Here's how the part is built. I have some questions about the finished solid (model axes, mm). A direction names the side the tool comes from. Round coordinates to 2 decimals unless told otherwise and drop trailing zeros. Order: outer loops, then holes, each group sorted by start corner. A loop starts at its lowest first (then second) coordinate and runs counter-clockwise, first axis right, second up. Notation, with made-up numbers: (-31, 22) -> (7, 22) arc R22 cw to (7, 42) -> close; hole circle Ø6 at (-31.5, 86.5). An arc over 180 degrees is marked (long way). One line per item, written item: value.
```python
from build123d import *

# Parameters (mm, degrees)
EXTRUDE1_DEPTH       = 39.5
SKETCH2_W            = 19.5
SKETCH2_H            = 8.1
EXTRUDE2_DEPTH       = 40.5
HOLEWZD1_D           = 8
HOLEWZD1_DEPTH       = 80.000025
HOLEWZD2_D           = 6.5
HOLEWZD2_CBORE_D     = 11
HOLEWZD2_CBORE_DEPTH = 4.4
FILLET1_R            = 1
FILLET2_R            = 3


with BuildPart() as part:
    # Sketch1 → Extrude1 (new body)
    with BuildSketch(Plane.XZ.offset(40)):
        with BuildLine():
            Line((-2, -8.1), (-2, -7.228416147))
            ThreePointArc((-2, -7.228416147), (5.968668193, 4.541475531), (-7.5, 0))
            Line((-7.5, 0), (-27.5, 0))
            Line((-27.5, 0), (-27.5, -8.1))
            Line((-27.5, -8.1), (-2, -8.1))
        make_face()
    extrude(amount=-EXTRUDE1_DEPTH)

    # Sketch2 → Extrude2 (add)
    with BuildSketch(Plane(origin=(0, -0.5, 0), x_dir=(-1, 0, 0), z_dir=(0, 1, 0))):
        with Locations((17.75, -4.05)):
            Rectangle(SKETCH2_W, SKETCH2_H)
    extrude(amount=EXTRUDE2_DEPTH)

    # HoleWzd1
    with Locations(Plane(origin=(0, -40, 0), x_dir=(-1, 0, 0), z_dir=(0, -1, 0))):
        with Locations((0, 0)):
            Hole(HOLEWZD1_D / 2, depth=HOLEWZD1_DEPTH)

    # HoleWzd2 (through all)
    with Locations(Plane.XY):
        with Locations((-15.5, -21.5), (-15.5, 21.5)):
            CounterBoreHole(HOLEWZD2_D / 2, HOLEWZD2_CBORE_D / 2, HOLEWZD2_CBORE_DEPTH)

    # Fillet1
    fillet1_edges = [part.edges().sort_by_distance(p)[0] for p in [
        (-27.5, 0, 0),
    ]]
    fillet(fillet1_edges, radius=FILLET1_R)

    # Fillet2
    # the kernel refuses this fillet: 3 mm, written as the material it takes off along each edge
    with BuildSketch(Plane(origin=(-27.5, -40, 6.5), x_dir=(1, 0, 0), z_dir=(0, 0, -1)), Plane(origin=(-27.5, 40, 6.5), x_dir=(0, -1, 0), z_dir=(0, 0, -1))) as fillet2_piece_1:
        with BuildLine():
            CenterArc((FILLET2_R, -FILLET2_R), FILLET2_R, 90, 90)
            Line((0, -FILLET2_R), (0, 0))
            Line((0, 0), (FILLET2_R, 0))
        make_face()
    extrude(amount=22.1, mode=Mode.SUBTRACT)


solid = part.part
```
Q1. Which directions (+Z, -Z, +X, -X, +Y, -Y) give clear straight access to the entire face, cutting with the end or side of a thin tool? Please do faces 1 (the face through (-12.543, 26.138, -2.169)), 2 (the face through (-8, 19, -4)), 3 (the face through (-17, -1, 0)), 4 (the face through (-16, 40, -4)).
Answers:
face 1: +Z
face 2: +Z, -Z, +X, +Y
face 3: +Z, -X, +Y, -Y
face 4: +Z, -Z, +X, -X, +Y
Q2. For P1, Ø1.5, axis at x = -20.5, y = 5.5, coming from the +Z side; P2, Ø3, axis at y = -15.5, z = 3.5, coming from the -X side; P3, Ø6, axis at x = -15.5, y = -21.5, coming from the +Z side; P4, Ø5.5, axis at x = -14.5, y = -24, coming from the +Z side, each with a flat end and sliding along its axis, tell me the tip position at first contact or that it passes through.
Answers:
P1: z = 0
P2: x = -7.23
P3: through
P4: z = -4.4
Q3. I need wall thicknesses on line 1 along Y through (x, z) = (-15.5, -2.95); line 2 along Z through (x, y) = (-11.5, -34.5); line 3 along Y through (x, z) = (-17.5, -6.25). Which ranges of each line are inside material? Lowest first, please.
Answers:
line 1: -40 to -27, -16 to 16, 27 to 40
line 2: -8.1 to 0
line 3: -40 to -24.06, -18.94 to 18.94, 24.06 to 40
Q4. I want a section at D-D on y = 21.5. Write out the boundary of the cut face in (x, z).
Answers:
outline: (-27.5, -8.1) -> (-18.75, -8.1) -> (-18.75, -4.4) -> (-21, -4.4) -> (-21, 0) -> (-26.5, 0) arc R1 ccw to (-27.5, -1) -> close; (-12.25, -8.1) -> (-8, -8.1) -> (-8, 0) -> (-10, 0) -> (-10, -4.4) -> (-12.25, -4.4) -> close
Q5. I want a section at C-C on z = -2.25. Write out the boundary of the cut face in (x, y).
Answers:
outline: (-27.5, -37) arc R3 ccw to (-24.5, -40) -> (-3.31, -40) -> (-3.31, -0.5) -> (-8, -0.5) -> (-8, 40) -> (-24.5, 40) arc R3 ccw to (-27.5, 37) -> close; (3.31, -40) -> (7.15, -40) -> (7.15, -0.5) -> (3.31, -0.5) -> close; hole circle Ø11 at (-15.5, -21.5); hole circle Ø11 at (-15.5, 21.5)
Q6. I want a section at A-A on y = -21.5. Write out the boundary of the cut face in (x, z), then the cut area to 3 significant figures.
Answers:
outline: (-27.5, -8.1) -> (-18.75, -8.1) -> (-18.75, -4.4) -> (-21, -4.4) -> (-21, 0) -> (-26.5, 0) arc R1 ccw to (-27.5, -1) -> close; (-12.25, -8.1) -> (-2, -8.1) -> (-2, -7.23) arc R7.5 ccw (long way) to (-7.5, 0) -> (-10, 0) -> (-10, -4.4) -> (-12.25, -4.4) -> close; hole circle Ø8 at (0, 0)
area: 231 mm2
Q7. I want a section at B-B on x = -15.5. Write out the boundary of the cut face in (y, z).
Answers:
outline: (-40, -8.1) -> (-24.75, -8.1) -> (-24.75, -4.4) -> (-27, -4.4) -> (-27, 0) -> (-40, 0) -> close; (-18.25, -8.1) -> (18.25, -8.1) -> (18.25, -4.4) -> (16, -4.4) -> (16, 0) -> (-16, 0) -> (-16, -4.4) -> (-18.25, -4.4) -> close; (24.75, -8.1) -> (40, -8.1) -> (40, 0) -> (27, 0) -> (27, -4.4) -> (24.75, -4.4) -> close
Q8. If we mould it in two halves opening along Y, with no side actions, what happens to faces 5 (the face through (-9, -40, -2)), 6 (the face through (-12.253, -21.357, -6.276)), 7 (the face through (-15, -1, -8.1))? For each: pulls with the +Y half, pulls with the -Y half, needs draft (parallel to the pull), parting line crosses it, or undercut.
Answers:
face 5: pulls with the -Y half
face 6: undercut
face 7: needs draft
